from build123d import *

# Parameters (mm, degrees)
SKETCH_1_W             = 203
SKETCH_1_H             = 37
SM_BASE_FLANGE_1_DEPTH = 5
FILLET_1_R             = 10
CUT_EXTRUDE_1_DEPTH    = 10
CUT_EXTRUDE_2_DEPTH    = 10
HOLE_WIZARD_M5_1_D     = 4.2
HOLE_WIZARD_M5_1_DEPTH = 12.4
HOLE_WIZARD_M5_1_TIP   = 1.2618073


# Sheet-metal steps are written as plain solids
with BuildPart() as part:
    # Sketch 1 → 基体-法兰1 (new body)
    with BuildSketch(Plane.XY):
        Rectangle(SKETCH_1_W, SKETCH_1_H)
    extrude(amount=-SM_BASE_FLANGE_1_DEPTH)

    # 圆角1
    fillet_1_edges = [part.edges().sort_by_distance(p)[0] for p in [
        (101.5, -18.5, -2.5),
        (-101.5, -18.5, -2.5),
        (-101.5, 18.5, -2.5),
        (101.5, 18.5, -2.5),
    ]]
    fillet(fillet_1_edges, radius=FILLET_1_R)

    # Sketch 2 → 切除-拉伸1 (cut)
    with BuildSketch(Plane(origin=(0, 0, -5), x_dir=(-1, 0, 0), z_dir=(0, 0, -1))):
        with BuildLine():
            Line((-58.5, -14), (-70.5, -14))
            ThreePointArc((-70.5, -14), (-84.5, 0), (-70.5, 14))
            Line((-70.5, 14), (-58.5, 14))
            ThreePointArc((-58.5, 14), (-44.5, 0), (-58.5, -14))
        make_face()
    extrude(amount=-CUT_EXTRUDE_1_DEPTH, mode=Mode.SUBTRACT)

    # 草图3 → 切除-拉伸2 (cut)
    with BuildSketch(Plane(origin=(0, 0, -5), x_dir=(-1, 0, 0), z_dir=(0, 0, -1))):
        with BuildLine():
            Line((60.5, -13), (52.5, -13))
            ThreePointArc((52.5, -13), (49.5, -10), (52.5, -7))
            Line((52.5, -7), (60.5, -7))
            ThreePointArc((60.5, -7), (63.5, -10), (60.5, -13))
        make_face()
        with BuildLine():
            Line((60.5, 7), (52.5, 7))
            ThreePointArc((52.5, 7), (49.5, 10), (52.5, 13))
            Line((52.5, 13), (60.5, 13))
            ThreePointArc((60.5, 13), (63.5, 10), (60.5, 7))
        make_face()
        with BuildLine():
            Line((82.5, 13), (90.5, 13))
            ThreePointArc((90.5, 13), (93.5, 10), (90.5, 7))
            Line((90.5, 7), (82.5, 7))
            ThreePointArc((82.5, 7), (79.5, 10), (82.5, 13))
        make_face()
        with BuildLine():
            Line((82.5, -7), (90.5, -7))
            ThreePointArc((90.5, -7), (93.5, -10), (90.5, -13))
            Line((90.5, -13), (82.5, -13))
            ThreePointArc((82.5, -13), (79.5, -10), (82.5, -7))
        make_face()
    extrude(amount=-CUT_EXTRUDE_2_DEPTH, mode=Mode.SUBTRACT)

    # M5 螺纹孔1
    with Locations(Plane(origin=(0, 0, -5), x_dir=(-1, 0, 0), z_dir=(0, 0, -1))):
        with Locations((-96.75, -7.9995), (-96.75, 8.0005), (-32.25, 8.0005), (-32.25, -7.9995)):
            Hole(HOLE_WIZARD_M5_1_D / 2, depth=HOLE_WIZARD_M5_1_DEPTH)
            with Locations((0, 0, -(HOLE_WIZARD_M5_1_DEPTH + HOLE_WIZARD_M5_1_TIP / 2))):  # 118° drill point
                Cone(0, HOLE_WIZARD_M5_1_D / 2, HOLE_WIZARD_M5_1_TIP, mode=Mode.SUBTRACT)


solid = part.part
The model under review builds one solid part; all positions refer to its coordinate system, in mm. A direction names the side the tool comes from. Coordinates: 2 decimals unless noted, no trailing zeros. Write each loop counter-clockwise with the first axis right and the second up, starting at its lowest first coordinate (ties: lowest second). Pieces come first, ordered by that corner, then holes. Notation, with made-up numbers: (68.5, -22) -> (110.5, -22) arc R30 cw to (110.5, 2) -> close; hole circle Ø1 at (7.25, 10). An arc over 180 degrees is marked (long way). Answer in a Markdown table with one row per item.
1. For faces 4 (the cylindrical face through (-98.65, 15.49, -2.54)), 5 (the flat face through (-57, -13, -3)), list the 3-axis set-ups (+Z, -Z, +X, -X, +Y, -Y) from which the entire face can be reached by the end or side of a thin tool; tool diameter is ignored.
Answers below:
| item | result |
|---|---|
| face 4 | +Z, -Z, -X, +Y |
| face 5 | +Z, -Z |
2. Wall thickness on probe 1 along Y at (x, z) = (32.25, -2.1); probe 2 along Y at (x, z) = (65, -2.85); probe 3 along Y at (x, z) = (-82, -0.75): over which ranges is each line inside the solid? List them lowest first. Write a range as [from, to].
Answers below:
| item | result |
|---|---|
| probe 1 | y = [-18.5, -10.1], [-5.9, 5.9], [10.1, 18.5] |
| probe 2 | y = [-18.5, -14], [14, 18.5] |
| probe 3 | y = [-18.5, -12.96], [-7.04, 7.04], [12.96, 18.5] |
3. We need section D-D, the plane x = 96.75. State the section outline as (y, z) points, and give its area (3 significant figures).
Answers below:
| item | result |
|---|---|
| outline | (-17.01, -5) -> (-10.1, -5) -> (-10.1, 0) -> (-17.01, 0) -> close; (-5.9, -5) -> (5.9, -5) -> (5.9, 0) -> (-5.9, 0) -> close; (10.1, -5) -> (17.01, -5) -> (17.01, 0) -> (10.1, 0) -> close |
| area | 128 mm^2 |
4. Draft analysis for pull direction Y (two halves, no side actions). For faces 1 (the flat face through (-1, -18.5, -2)), 2 (the cylindrical face through (-63.5, 10.1, -2.5)), 3 (the flat face through (-1, 18.5, -2)), state which applies: +Y half, -Y half, draft (parallel to the pull), parting line (faces both ways), or undercut.
Answers below:
| item | result |
|---|---|
| face 1 | -Y half |
| face 2 | undercut |
| face 3 | +Y half |
5. We need section B-B, the plane x = 32.25. State the section outline as (y, z) points.
Answers below:
| item | result |
|---|---|
| outline | (-18.5, -5) -> (-10.1, -5) -> (-10.1, 0) -> (-18.5, 0) -> close; (-5.9, -5) -> (5.9, -5) -> (5.9, 0) -> (-5.9, 0) -> close; (10.1, -5) -> (18.5, -5) -> (18.5, 0) -> (10.1, 0) -> close |
6. Clearance check with a flat-ended pin moving along its axis: pin 1 Ø4 at (x, y) = (32.25, -8) entering from +Z. State where the tip first meets the part, or that it passes through.
Answers below:
| item | result |
|---|---|
| pin 1 | passes through |
7. We need section A-A, the plane y = 0. State the section outline as (x, z) points, and give its area (3 significant figures).
Answers below:
| item | result |
|---|---|
| outline | (-101.5, -5) -> (44.5, -5) -> (44.5, 0) -> (-101.5, 0) -> close; (84.5, -5) -> (101.5, -5) -> (101.5, 0) -> (84.5, 0) -> close |
| area | 815 mm^2 |
8. We need section C-C, the plane z = -1. Give the number of separate pieces and of enclosed holes in the cut face, and give its area (3 significant figures).
Answers below:
| item | result |
|---|---|
| separate pieces | 1 |
| enclosed holes | 9 |
| area | 6,110 mm^2 |
